Autodesk Inventor part; units mm, degrees
ref_plane "YZ Plane" through (0, 0, 0) normal (1, 0, 0) x (0, 1, 0)
ref_plane "XZ Plane" through (0, 0, 0) normal (0, 1, 0) x (-1, 0, 0)
ref_plane "XY Plane" through (0, 0, 0) normal (0, 0, 1) x (1, 0, 0)
sketch "Sketch1" plane through (0, 0, 0) normal (0, 0, 1) x (1, 0, 0)
  circle A0 centre (0, 0) radius 125
  circle A1 centre (0, 0) radius 164.5
  dimension "d0" = 39.5
  dimension "d1" = 250
extrude "Extrusion1" add sketch "Sketch1" along normal blind 41
sketch "Sketch2" plane through (0, 0, 41) normal (0, 0, 1) x (1, 0, 0)
  circle A0 centre (0, 0) radius 164.5 construction
  circle A1 centre (0, 0) radius 125 construction
  line L0 (0, 164.5) -> (0, 125) construction
  circle A2 centre (0, 144.75) radius 6.25
  dimension "d4" = 12.5
extrude "Extrusion2" cut sketch "Sketch2" against normal through all
sketch "Sketch3" plane through (0, 0, 41) normal (0, 0, 1) x (1, 0, 0)
  circle A0 centre (0, 144.75) radius 6.25
  circle A1 centre (0, 144.75) radius 13.75
  point P0 (0, 0)
  dimension "d10" = 27.5
extrude "Extrusion3" cut sketch "Sketch3" against normal blind 11
pattern_circular "Circular Pattern1" count 8 over 360 about axis through (0, 0, 0) along (0, 0, 1) of "Extrusion2", "Extrusion3"
sketch "Sketch4" plane through (0, 0, 0) normal (0, 0, -1) x (-1, 0, 0)
  circle A0 centre (0, 0) radius 164.5
  circle A1 centre (0, 0) radius 169.5
  dimension "d13" = 5
extrude "Extrusion4" add sketch "Sketch4" against normal blind 10
equation "\"d1\" = Вал_ось_диаметр_НОС"
properties part number "ДМФ 01 31 Барабан Опорное кольцо НОС v2.0"
CAD build for the part. Positions are in the model's coordinates, mm. A direction names the side the tool comes from. Round coordinates to 2 decimals unless told otherwise and drop trailing zeros. Loops run counter-clockwise (first coordinate to the right, second up) from the corner with the lowest first, then second, coordinate; pieces in that order, holes last. Notation, with made-up numbers: M -15,29 L 4,29 A18 ccw 4,36 Z; hole C 78.25,-36 d4. An arc over 180 degrees is marked long. Use a Markdown table: item, result. Add a question column.
(1) Which spindle directions (+Z, -Z, +X, -X, +Y, -Y) get a long thin tool onto all of the face, cutting with end or side? Do faces 1 (the face through (-96, 100, 30)), 2 (the face through (-2.884, -139.205, 15.21)). Say none if no direction does.
(2) Drill centre lines: line 1 (Y direction, x = -1, z = 22.5); line 2 (Y direction, x = 0, z = 14); line 3 (X direction, y = 98, z = 32). Where is each one in solid material? Low to high.
(3) Cut at A-A (y = 0). Give the cut face in (x, z).
(4) Pull direction X, two halves, no side cores. Call faces 3 (the face through (89, 89, 0)), 4 (the face through (36.74, -165.47, 4.93)), 5 (the face through (139.205, -2.884, 15.21)): +X half, -X half, draft (parallel to the pull), parting line (faces both ways), or undercut.
(5) Cut at D-D (x = -45). Give the cut face in (y, z), and give its area (3 significant figures).
(6) Flat gauge pins, fed straight in: pin 1 (16.5 mm diameter, centred on x = -102.35, y = -102.35, fed in from +Z); pin 2 (4 mm diameter, centred on y = -110, z = 10.5, fed in from -X); pin 3 (2 mm diameter, centred on y = -81.5, z = 10.5, fed in from -X). Where does each tip first touch, or does it go through?
Geometry says:
| question | item | result |
|---|---|---|
| 1 | face 1 | +Z |
| 1 | face 2 | +Z, -Z |
| 2 | line 1 | y = -164.5 to -150.92, -138.58 to -125, 125 to 138.58, 150.92 to 164.5 |
| 2 | line 2 | y = -164.5 to -151, -138.5 to -125, 125 to 138.5, 151 to 164.5 |
| 2 | line 3 | x = -132.12 to -115.4, -89.31 to -77.6, 77.6 to 89.31, 115.4 to 132.12 |
| 3 | outline | M -169.5,0 L -151,0 L -151,30 L -158.5,30 L -158.5,41 L -164.5,41 L -164.5,10 L -169.5,10 Z; M -138.5,0 L -125,0 L -125,41 L -131,41 L -131,30 L -138.5,30 Z; M 125,0 L 138.5,0 L 138.5,30 L 131,30 L 131,41 L 125,41 Z; M 151,0 L 169.5,0 L 169.5,10 L 164.5,10 L 164.5,41 L 158.5,41 L 158.5,30 L 151,30 Z |
| 4 | face 3 | draft |
| 4 | face 4 | parting line |
| 4 | face 5 | undercut |
| 5 | outline | M -163.42,0 L -116.62,0 L -116.62,41 L -158.23,41 L -158.23,10 L -163.42,10 Z; M 116.62,0 L 163.42,0 L 163.42,10 L 158.23,10 L 158.23,41 L 116.62,41 Z |
| 5 | area | 3,520 mm² |
| 6 | pin 1 | stops at z = 30 |
| 6 | pin 2 | stops at x = -130.59 |
| 6 | pin 3 | stops at x = -149.09 |
